Autodesk Fusion 360 part; units mm, degrees
sketch "Sketch1" plane through (0, 0, 0) normal (0, 0, 1) x (1, 0, 0)
  line L0 (40.5, 29) -> (-40.5, 29)
  line L1 (-40.5, 29) -> (-40.5, -29)
  line L2 (-40.5, -29) -> (40.5, -29)
  line L3 (40.5, -29) -> (40.5, 29)
  line L4 (40.5, 29) -> (-40.5, -29) construction
  line L5 (-40.5, 29) -> (40.5, -29) construction
  dimension "d1" = 81
  dimension "d2" = 58
extrude "Extrude1" add sketch "Sketch1" along normal blind 22.5
sketch "Sketch2" plane through (0, 0, 22.5) normal (0, 0, 1) x (-1, 0, 0)
  line L0 (-40.5, 29) -> (-40.5, -29)
  line L1 (-40.5, -29) -> (40.5, -29)
  line L2 (40.5, -29) -> (40.5, 29)
  line L3 (40.5, 29) -> (-40.5, 29)
  line L4 (-37.5, -26) -> (37.5, -26)
  line L5 (37.5, -26) -> (37.5, 26)
  line L6 (37.5, 26) -> (-37.5, 26)
  line L7 (-37.5, 26) -> (-37.5, -26)
  line L8 (-37.5, -26) -> (37.5, 26) construction
  line L9 (37.5, -26) -> (-37.5, 26) construction
  dimension "d5" = 75
  dimension "d6" = 52
extrude "Extrude2" cut sketch "Sketch2" against normal blind 19.5 contours L4 L5 L6 L7
sketch "Sketch3" plane through (0, 0, 0) normal (0, 0, -1) x (1, 0, 0)
  line L0 (40.5, -29) -> (40.5, 29)
  line L1 (40.5, 29) -> (-40.5, 29)
  line L2 (-40.5, 29) -> (-40.5, -29)
  line L3 (-40.5, -29) -> (40.5, -29)
  line L4 (33.25, 21.75) -> (-33.25, 21.75)
  line L5 (-33.25, 21.75) -> (-33.25, -21.75)
  line L6 (-33.25, -21.75) -> (33.25, -21.75)
  line L7 (33.25, -21.75) -> (33.25, 21.75)
  line L8 (33.25, 21.75) -> (-33.25, -21.75) construction
  line L9 (-33.25, 21.75) -> (33.25, -21.75) construction
  dimension "d9" = 66.5
  dimension "d10" = 43.5
sketch "Sketch4" plane through (0, 0, 0) normal (0, 0, -1) x (1, 0, 0)
extrude "Extrude3" cut sketch "Sketch3" against normal blind 3 contours L4 L5 L6 L7
sketch "Sketch5" plane through (0, 0, 3) normal (0, 0, 1) x (-1, 0, 0)
  line L0 (-33.25, 21.75) -> (33.25, 21.75)
  line L1 (33.25, 21.75) -> (33.25, -21.75)
  line L2 (33.25, -21.75) -> (-33.25, -21.75)
  line L3 (-33.25, -21.75) -> (-33.25, 21.75)
  line L4 (-37.5, 26) -> (-37.5, -26)
  line L5 (-37.5, -26) -> (37.5, -26)
  line L6 (37.5, -26) -> (37.5, 26)
  line L7 (37.5, 26) -> (-37.5, 26)
  circle A0 centre (35.875, -24.375) radius 1.5
  dimension "d13" = 3
  dimension "d14" = 1.625
  dimension "d15" = 1.625
sketch "Sketch6" plane through (0, 0, 3) normal (0, 0, 1) x (-1, 0, 0)
  circle A0 centre (-35.875, -24.375) radius 1.5
  line L0 (-37.5, -26) -> (37.5, -26)
  line L1 (-37.5, 26) -> (-37.5, -26)
  circle A1 centre (-35.875, 24.375) radius 1.5
  line L2 (37.5, 26) -> (-37.5, 26)
  circle A2 centre (35.875, 24.375) radius 1.5
  line L3 (37.5, -26) -> (37.5, 26)
  dimension "d16" = 3
  dimension "d17" = 1.625
  dimension "d18" = 1.625
  dimension "d19" = 3
  dimension "d20" = 1.625
  dimension "d21" = 1.625
  dimension "d25" = 3
  dimension "d26" = 1.625
  dimension "d27" = 1.625
sketch "Sketch8" plane through (0, -29, 0) normal (0, -1, 0) x (1, 0, 0)
  line L0 (-40.5, 0) -> (40.5, 0)
  line L1 (40.5, 0) -> (40.5, 22.5)
  line L2 (40.5, 22.5) -> (-40.5, 22.5)
  line L3 (-40.5, 22.5) -> (-40.5, 0)
  line L4 (31.5, 15) -> (-31.5, 15)
  line L5 (-31.5, 15) -> (-31.5, 5)
  line L6 (-31.5, 5) -> (31.5, 5)
  line L7 (31.5, 5) -> (31.5, 15)
  line L8 (31.5, 15) -> (-31.5, 5) construction
  line L9 (-31.5, 15) -> (31.5, 5) construction
  point P0 (0, 10)
  dimension "d30" = 63
  dimension "d31" = 10
  dimension "d33" = 15
extrude "Extrude5" cut sketch "Sketch8" against normal blind 3 contours L4 L5 L6 L7
sketch "Sketch9" plane through (0, 29, 0) normal (0, 1, 0) x (-1, 0, 0)
  line L0 (-40.5, 0) -> (40.5, 0)
  line L1 (40.5, 0) -> (40.5, 22.5)
  line L2 (40.5, 22.5) -> (-40.5, 22.5)
  line L3 (-40.5, 22.5) -> (-40.5, 0)
  line L4 (32.5, 15) -> (2.5, 15)
  line L5 (2.5, 15) -> (2.5, 5)
  line L6 (2.5, 5) -> (32.5, 5)
  line L7 (32.5, 5) -> (32.5, 15)
  line L8 (32.5, 15) -> (2.5, 5) construction
  line L9 (2.5, 15) -> (32.5, 5) construction
  point P0 (17.5, 10)
  dimension "d36" = 30
  dimension "d37" = 10
  dimension "d38" = 8
  dimension "d39" = 15
extrude "Extrude6" cut sketch "Sketch9" against normal blind 3 contours L4 L5 L6 L7
sketch "Sketch11" plane through (0, 0, 22.5) normal (0, 0, 1) x (-1, 0, 0)
  line L0 (37.5, -26) -> (-37.5, -26)
  line L1 (-37.5, -26) -> (-37.5, 26)
  line L2 (-37.5, 26) -> (37.5, 26)
  line L3 (37.5, 26) -> (37.5, -26)
  line L4 (-40.5, 29) -> (-40.5, -29)
  line L5 (-40.5, -29) -> (40.5, -29)
  line L6 (40.5, -29) -> (40.5, 29)
  line L7 (40.5, 29) -> (-40.5, 29)
  circle A0 centre (38.375, -26.875) radius 1
  circle A1 centre (38.375, 26.875) radius 1
  circle A2 centre (-38.375, 26.875) radius 1
  circle A3 centre (-38.375, -26.875) radius 1
  dimension "d56" = 2
  dimension "d57" = 2
  dimension "d58" = 2
  dimension "d59" = 2
  dimension "d60" = 2.125
  dimension "d61" = 2.125
  dimension "d62" = 2.125
  dimension "d63" = 2.125
  dimension "d64" = 2.125
  dimension "d65" = 2.125
  dimension "d66" = 2.125
  dimension "d67" = 2.125
hole "Hole1" at (-38.375, 26.875, 22.5) at (38.375, 26.875, 22.5) at (38.375, -26.875, 22.5) at (-38.375, -26.875, 22.5) direction (0, 0, -1) diameter 1.6256 depth 5 tip angle 180
sketch "Sketch12" plane through (0, 0, 0) normal (0, 0, 1) x (1, 0, 0)
sketch "Sketch13" plane through (0, 0, 3) normal (0, 0, 1) x (-1, 0, 0)
  line L0 (-33.25, 21.75) -> (33.25, 21.75)
  line L1 (33.25, 21.75) -> (33.25, -21.75)
  line L2 (33.25, -21.75) -> (-33.25, -21.75)
  line L3 (-33.25, -21.75) -> (-33.25, 21.75)
  line L4 (-37.5, 26) -> (-37.5, -26)
  line L5 (-37.5, -26) -> (37.5, -26)
  line L6 (37.5, -26) -> (37.5, 26)
  line L7 (37.5, 26) -> (-37.5, 26)
  circle A0 centre (33, 21.5) radius 1.25
  dimension "d73" = 2.5
  dimension "d74" = 4.5
  dimension "d75" = 4.5
sketch "Sketch14" plane through (0, 0, 3) normal (0, 0, 1) x (-1, 0, 0)
Read the model definition and answer for the solid it produces. Units are mm, in the model's axes. A direction names the side the tool comes from. Round coordinates to 2 decimals unless told otherwise and drop trailing zeros. Write each loop counter-clockwise with the first axis right and the second up, starting at its lowest first coordinate (ties: lowest second). Pieces come first, ordered by that corner, then holes. Notation, with made-up numbers: M 5.25,-2.5 L 19.25,-2.5 A21 cw 19.25,36.5 Z; hole C 38.25,76.5 d11. An arc over 180 degrees is marked long. Use a Markdown table: item, result.
1) A tool of negligible diameter and unlimited length cuts with its end or side. For faces 4 (the flat face through (31.5, -28, 10)), 5 (the flat face through (-33.25, 0, 1)), 6 (the cylindrical face through (-37.88, 27.52, 19.96)), from which of +Z, -Z, +X, -X, +Y, -Y can it reach the whole face along a straight path? Write none if from no direction.
Answers follow:
| item | result |
|---|---|
| face 4 | -Y |
| face 5 | +Z, -Z |
| face 6 | +Z |
2) Flat-ended cylindrical pins translate along their axes: pin 1 (4 mm diameter, centred on x = -31.5, y = -4, fed in from +Z); pin 2 (1 mm diameter, centred on x = 38.375, y = -26.875, fed in from -Z). Find the tip coordinate at first contact, or state that the pin passes through.
Answers follow:
| item | result |
|---|---|
| pin 1 | stops at z = 3 |
| pin 2 | stops at z = 0 |
3) The part is cut by section C-C (z = 6). Write down the section's boundary in (x, y).
Answers follow:
| item | result |
|---|---|
| outline | M -40.5,-29 L -31.5,-29 L -31.5,-26 L -37.5,-26 L -37.5,26 L -32.5,26 L -32.5,29 L -40.5,29 Z; M -2.5,26 L 37.5,26 L 37.5,-26 L 31.5,-26 L 31.5,-29 L 40.5,-29 L 40.5,29 L -2.5,29 Z |
4) The part is cut by section B-B (x = -10). Write down the section's boundary in (y, z).
Answers follow:
| item | result |
|---|---|
| outline | M -29,0 L -21.75,0 L -21.75,3 L -26,3 L -26,5 L -29,5 Z; M -29,15 L -26,15 L -26,22.5 L -29,22.5 Z; M 21.75,0 L 29,0 L 29,5 L 26,5 L 26,3 L 21.75,3 Z; M 26,15 L 29,15 L 29,22.5 L 26,22.5 Z |
5) The part is cut by section A-A (y = 2). Write down the section's boundary in (x, z).
Answers follow:
| item | result |
|---|---|
| outline | M -40.5,0 L -33.25,0 L -33.25,3 L -37.5,3 L -37.5,22.5 L -40.5,22.5 Z; M 33.25,0 L 40.5,0 L 40.5,22.5 L 37.5,22.5 L 37.5,3 L 33.25,3 Z |
6) For a pull along Z with two mould halves and no side action, classify faces 1 (the flat face through (-38, 27, 17.5)), 2 (the flat face through (33.25, 0, 1)), 3 (the flat face through (-2.5, 28, 10)) as pulls with the +Z half, pulls with the -Z half, needs draft (parallel to the pull), parting line crosses it, or undercut.
Answers follow:
| item | result |
|---|---|
| face 1 | pulls with the +Z half |
| face 2 | needs draft |
| face 3 | undercut |
7) The part is cut by section D-D (x = 25.5). Write down the section's boundary in (y, z).
Answers follow:
| item | result |
|---|---|
| outline | M -29,0 L -21.75,0 L -21.75,3 L -26,3 L -26,5 L -29,5 Z; M -29,15 L -26,15 L -26,22.5 L -29,22.5 Z; M 21.75,0 L 29,0 L 29,22.5 L 26,22.5 L 26,3 L 21.75,3 Z |
8) Straight lines are drawn through the part: line 1 along Y through (x, z) = (36, 16.5); line 2 along X through (y, z) = (11.5, 17.5); line 3 along Y through (x, z) = (-10, 1.75). For each, find the intervals that lie inside material, in ascending order. Write a range as [from, to].
Answers follow:
| item | result |
|---|---|
| line 1 | y = [-29, -26], [26, 29] |
| line 2 | x = [-40.5, -37.5], [37.5, 40.5] |
| line 3 | y = [-29, -21.75], [21.75, 29] |
